from build123d import *

# Parameters (mm, degrees)
F0_W           = 889
F0_H           = 889
F1_DEPTH       = 25.4
F6_DEPTH       = 12.7
F3_D           = 3.175
F3_DEPTH       = 63.5
F3_CBORE_D     = 12.7
F3_CBORE_DEPTH = 3.175
F4_R           = 127


with BuildPart() as f1:
    # F0 (on Top) → F1 (new body)
    with BuildSketch(Plane.XY):
        Rectangle(F0_W, F0_H)
    extrude(amount=F1_DEPTH)

    # F5 (on face) → F6 (cut)
    with BuildSketch(Plane.XY.offset(25.4)):
        Polygon((12.7, 12.7), (12.7, 254), (-12.7, 254), (-12.7, 12.7), (-254, 12.7), (-254, -12.7), (-12.7, -12.7), (-12.7, -254), (12.7, -254), (12.7, -12.7), (254, -12.7), (254, 12.7), align=None)
    extrude(amount=-F6_DEPTH, mode=Mode.SUBTRACT)

    # F3
    with Locations(Plane(origin=(0, 0, 0), x_dir=(1, 0, 0), z_dir=(0, 0, -1))):
        with Locations((-190.5, 0), (0, 190.5), (190.5, 0), (0, -190.5)):
            CounterBoreHole(F3_D / 2, F3_CBORE_D / 2, F3_CBORE_DEPTH, depth=F3_DEPTH)

    # F4
    f4_edges = [f1.edges().sort_by_distance(p)[0] for p in [
        (444.5, -444.5, 12.7),
        (444.5, 444.5, 12.7),
        (-444.5, 444.5, 12.7),
        (-444.5, -444.5, 12.7),
    ]]
    fillet(f4_edges, radius=F4_R)


solid = f1.part
The model under review builds one solid part; all positions refer to its coordinate system, in mm. Round coordinates to 2 decimals unless told otherwise and drop trailing zeros. Loops run counter-clockwise (first coordinate to the right, second up) from the corner with the lowest first, then second, coordinate; pieces in that order, holes last. Notation, with made-up numbers: (-34.5, 70.25) -> (9.5, 70.25) arc R11 cw to (9.5, 89.25) -> close; hole circle Ø8 at (74, 47.5). An arc over 180 degrees is marked (long way). Write item = value, one per line. Start each with the question number.
Item 1: To check wall thickness, follow L1, parallel to X at y = -136, z = 18.75; L2, parallel to Y at x = 190.5, z = 0.8. State the ranges of each line that lie inside material, in increasing order.
Item 2: Take a section at A-A on z = 8.75. Give the boundary of the cut face in (x, y) (1 decimal), plus the area to 3 significant figures.
Item 3: Mouldability with a two-part tool opening along Y and no side actions: class faces 1 (the flat face through (-444.5, -4, 13)), 2 (the cylindrical face through (406.31, -408.285, 12.878)), 3 (the cylindrical face through (-408.285, 406.31, 12.878)), 4 (the flat face through (-1, 1, 12.7)) as released by +Y, released by -Y, zero draft, split by the parting line, or undercut.
Item 4: Take a section at B-B on x = 361.5. Give the boundary of the cut face in (y, z), plus the area to 3 significant figures.
Item 5: Insertion check: pin 1 (3 mm diameter, centred on x = -330.5, z = 12.5, fed in from -Y); pin 2 (6.5 mm diameter, centred on x = -190, y = 2, fed in from -Z) (3 decimals); pin 3 (14.5 mm diameter, centred on x = 0, y = -190.5, fed in from +Z). Each pin has a flat end and moves straight along its axis. Give the tip position at first contact, or say it passes through.
Result:
q1.L1 = -444.5 to -12.7, 12.7 to 444.5
q1.L2 = -444.5 to -6.35, 6.35 to 444.5
q2.outline = (-444.5, -317.5) arc R127 ccw to (-317.5, -444.5) -> (317.5, -444.5) arc R127 ccw to (444.5, -317.5) -> (444.5, 317.5) arc R127 ccw to (317.5, 444.5) -> (-317.5, 444.5) arc R127 ccw to (-444.5, 317.5) -> close; hole circle Ø3.2 at (-190.5, 0); hole circle Ø3.2 at (0, -190.5); hole circle Ø3.2 at (0, 190.5); hole circle Ø3.2 at (190.5, 0)
q2.area = 776,000 mm²
q3.face_1 = zero draft
q3.face_2 = released by -Y
q3.face_3 = released by +Y
q3.face_4 = undercut
q4.outline = (-436.63, 0) -> (436.63, 0) -> (436.63, 25.4) -> (-436.63, 25.4) -> close
q4.area = 22,200 mm²
q5.pin_1 = -443.98
q5.pin_2 = 3.175
q5.pin_3 = 12.7
